```python
from build123d import *

# Parameters (mm, degrees)
SKETCH_1_W      = 48
SKETCH_1_H      = 48
SKETCH_1_R      = 1.55
SKETCH_1_R_2    = 1.6
SKETCH_1_R_3    = 1.65
SKETCH_1_R_4    = 1.7
SKETCH_1_R_5    = 1.75
EXTRUDE_1_DEPTH = 3


with BuildPart() as part:
    # 草图1 → 凸台-拉伸1 (new body)
    with BuildSketch(Plane.XY):
        with Locations((24, 24)):
            Rectangle(SKETCH_1_W, SKETCH_1_H)
        with Locations((8, 8)):
            Circle(SKETCH_1_R, mode=Mode.SUBTRACT)
        with Locations((8, 16)):
            Circle(SKETCH_1_R, mode=Mode.SUBTRACT)
        with Locations((8, 24)):
            Circle(SKETCH_1_R, mode=Mode.SUBTRACT)
        with Locations((8, 32)):
            Circle(SKETCH_1_R, mode=Mode.SUBTRACT)
        with Locations((8, 40)):
            Circle(SKETCH_1_R, mode=Mode.SUBTRACT)
        with Locations((16, 8)):
            Circle(SKETCH_1_R_2, mode=Mode.SUBTRACT)
        with Locations((16, 16)):
            Circle(SKETCH_1_R_2, mode=Mode.SUBTRACT)
        with Locations((16, 24)):
            Circle(SKETCH_1_R_2, mode=Mode.SUBTRACT)
        with Locations((16, 32)):
            Circle(SKETCH_1_R_2, mode=Mode.SUBTRACT)
        with Locations((16, 40)):
            Circle(SKETCH_1_R_2, mode=Mode.SUBTRACT)
        with Locations((24, 8)):
            Circle(SKETCH_1_R_3, mode=Mode.SUBTRACT)
        with Locations((24, 16)):
            Circle(SKETCH_1_R_3, mode=Mode.SUBTRACT)
        with Locations((24, 24)):
            Circle(SKETCH_1_R_3, mode=Mode.SUBTRACT)
        with Locations((24, 32)):
            Circle(SKETCH_1_R_3, mode=Mode.SUBTRACT)
        with Locations((24, 40)):
            Circle(SKETCH_1_R_3, mode=Mode.SUBTRACT)
        with Locations((32, 8)):
            Circle(SKETCH_1_R_4, mode=Mode.SUBTRACT)
        with Locations((32, 16)):
            Circle(SKETCH_1_R_4, mode=Mode.SUBTRACT)
        with Locations((32, 24)):
            Circle(SKETCH_1_R_4, mode=Mode.SUBTRACT)
        with Locations((32, 32)):
            Circle(SKETCH_1_R_4, mode=Mode.SUBTRACT)
        with Locations((32, 40)):
            Circle(SKETCH_1_R_4, mode=Mode.SUBTRACT)
        with Locations((40, 8)):
            Circle(SKETCH_1_R_5, mode=Mode.SUBTRACT)
        with Locations((40, 16)):
            Circle(SKETCH_1_R_5, mode=Mode.SUBTRACT)
        with Locations((40, 24)):
            Circle(SKETCH_1_R_5, mode=Mode.SUBTRACT)
        with Locations((40, 32)):
            Circle(SKETCH_1_R_5, mode=Mode.SUBTRACT)
        with Locations((40, 40)):
            Circle(SKETCH_1_R_5, mode=Mode.SUBTRACT)
    extrude(amount=EXTRUDE_1_DEPTH)


solid = part.part
```
For this review, take the finished solid that the model builds, in its own axes (mm). Coordinates: 2 decimals unless noted, no trailing zeros. Write each loop counter-clockwise with the first axis right and the second up, starting at its lowest first coordinate (ties: lowest second). Pieces come first, ordered by that corner, then holes. Notation, with made-up numbers: (6.5, 22.25) -> (62.5, 22.25) arc R15 cw to (62.5, 51.25) -> close; hole circle Ø10 at (-23, 47). An arc over 180 degrees is marked (long way). Put each result on its own line as item: value.
Q1. Take a section at A-A, the plane x = 8. State the section outline as (y, z) points.
From the geometry:
outline: (0, 0) -> (6.45, 0) -> (6.45, 3) -> (0, 3) -> close; (9.55, 0) -> (14.45, 0) -> (14.45, 3) -> (9.55, 3) -> close; (17.55, 0) -> (22.45, 0) -> (22.45, 3) -> (17.55, 3) -> close; (25.55, 0) -> (30.45, 0) -> (30.45, 3) -> (25.55, 3) -> close; (33.55, 0) -> (38.45, 0) -> (38.45, 3) -> (33.55, 3) -> close; (41.55, 0) -> (48, 0) -> (48, 3) -> (41.55, 3) -> close
Q2. The part is to be moulded in two halves that separate along X. For faces 1 (the flat face through (0, 24, 1)), 2 (the flat face through (24, 48, 1)), 3 (the cylindrical face through (41.617, 7.33, 1.479)), say which applies: +X half, -X half, draft (parallel to the pull), parting line (faces both ways), or undercut.
From the geometry:
face 1: -X half
face 2: draft
face 3: undercut
Q3. Take a section at B-B, the plane y = 40. State the section outline as (x, z) points.
From the geometry:
outline: (0, 0) -> (6.45, 0) -> (6.45, 3) -> (0, 3) -> close; (9.55, 0) -> (14.4, 0) -> (14.4, 3) -> (9.55, 3) -> close; (17.6, 0) -> (22.35, 0) -> (22.35, 3) -> (17.6, 3) -> close; (25.65, 0) -> (30.3, 0) -> (30.3, 3) -> (25.65, 3) -> close; (33.7, 0) -> (38.25, 0) -> (38.25, 3) -> (33.7, 3) -> close; (41.75, 0) -> (48, 0) -> (48, 3) -> (41.75, 3) -> close
Q4. Take a section at C-C, the plane z = 1.45. Count the separate pieces of the cut face and the enclosed holes in it, then the cut area to 3 significant figures.
From the geometry:
separate pieces: 1
enclosed holes: 25
area: 2,090 mm2
Q5. Clearance check with a flat-ended pin moving along its axis: pin 1 Ø2 at (x, y) = (40, 16) entering from -Z. State where the tip first meets the part, or that it passes through.
From the geometry:
pin 1: passes through
Q6. Wall thickness on L1, parallel to Y at x = 24, z = 2.25; L2, parallel to Y at x = 8, z = 2.3; L3, parallel to X at y = 24.5, z = 1.7: over which ranges is each line inside the solid? List them lowest first.
From the geometry:
L1: y = 0 to 6.35, 9.65 to 14.35, 17.65 to 22.35, 25.65 to 30.35, 33.65 to 38.35, 41.65 to 48
L2: y = 0 to 6.45, 9.55 to 14.45, 17.55 to 22.45, 25.55 to 30.45, 33.55 to 38.45, 41.55 to 48
L3: x = 0 to 6.53, 9.47 to 14.48, 17.52 to 22.43, 25.57 to 30.38, 33.62 to 38.32, 41.68 to 48
